Build history of the part. All positions in model axes, mm. A direction names the side the tool comes from. Give positions to 0.01 mm unless a question says otherwise; leave off trailing zeros. Order: outer loops, then holes, each group sorted by start corner. A loop starts at its lowest first (then second) coordinate and runs counter-clockwise, first axis right, second up. Notation, with made-up numbers: (42.25, 58) - (54.25, 58) arc R24 cw to (54.25, 84) - close; hole circle Ø2 at (-1, -33). An arc over 180 degrees is marked (long way). Write each question's results on one line, items separated by ' | '. Start each with the question number.
1) Cut at C-C on x = -892. List the corners of the cut face in (y, z), plus the area to 3 significant figures.
2) Cut at A-A on y = 344.5. List the corners of the cut face in (x, z).
3) Two-plate mould, pull along X, no slides. Class faces 1 (the face through (118.392, 25, -201)), 2 (the face through (650, 50, -277)), 3 (the face through (20, 50, -261)): +X half, -X half, draft (parallel to the pull), parting line (faces both ways), or undercut.
4) Drill centre lines: line 1 along X through (y, z) = (332.5, -290.5); line 2 along Y through (x, z) = (-757.5, -293); line 3 along X through (y, z) = (118.5, -263). Where is each one in solid material? Low to high. Write a range as from..to.
5) Drop flat-ended pins along their axis: pin 1 Ø12 at (x, z) = (9, -253.5) entering from +Y; pin 2 Ø6 at (y, z) = (21.5, -294) entering from +X; pin 3 Ø2 at (y, z) = (275, -258) entering from -X. Give the stop position or say it passes through.
6) Cut at B-B on z = -199.5. List the corners of the cut face in (x, y), plus the area to 3 significant figures.
7) Tool access for faces 4 (the face through (118.392, 272, -276)), 5 (the face through (-131.608, 272, -276)), 6 (the face through (168.392, 272, -276)), 7 (the face through (-81.608, 25, -202)), 8 (the face through (18, 25, -251.508)): list every direction of +Z, -Z, +X, -X, +Y, -Y with a clear straight run to the whole face (end or side of a thin tool).
from build123d import *

# Parameters (mm, degrees)
SKETCH1_W           = 20
SKETCH1_H           = 40
BOSS_EXTRUDE1_DEPTH = 50
SKETCH2_W           = 50
SKETCH2_H           = 50
BOSS_EXTRUDE2_DEPTH = 1000
SKETCH3_W           = 50
SKETCH3_H           = 50
BOSS_EXTRUDE3_DEPTH = 1000
SKETCH4_W           = 50
SKETCH4_H           = 50
BOSS_EXTRUDE4_DEPTH = 450
SKETCH6_W           = 650
SKETCH6_H           = 20
CUT_EXTRUDE2_DEPTH  = 20
SKETCH7_W           = 20
SKETCH7_H           = 450
CUT_EXTRUDE3_DEPTH  = 20


with BuildPart() as part:
    # Sketch1 → Boss-Extrude1 (new body)
    with BuildSketch(Plane(origin=(0, 0, 0), x_dir=(1, 0, 0), z_dir=(0, 1, 0))):
        Polygon((-31.607653806, 251.508316195), (0, 251.508316195), (68.392346194, 251.508316195), (68.392346194, 221.086115448), (68.392346194, 181.086115448), (68.392346194, 151.508316195), (118.392346194, 151.508316195), (118.392346194, 301.508316195), (-81.607653806, 301.508316195), (-81.607653806, 151.508316195), (-31.607653806, 151.508316195), (-31.607653806, 181.086115448), (-31.607653806, 221.086115448), align=None)
        with Locations((-21.607653806, 201.086115448)):
            Rectangle(SKETCH1_W, SKETCH1_H)
        with Locations((58.392346194, 201.086115448)):
            Rectangle(SKETCH1_W, SKETCH1_H)
    extrude(amount=BOSS_EXTRUDE1_DEPTH)

    # Sketch2 → Boss-Extrude2 (add)
    with BuildSketch(Plane(origin=(118.392346194, 0, 0), x_dir=(0, 0, -1), z_dir=(1, 0, 0))):
        with Locations((276.508316195, 25)):
            Rectangle(SKETCH2_W, SKETCH2_H)
    extrude(amount=BOSS_EXTRUDE2_DEPTH)

    # Sketch3 → Boss-Extrude3 (add)
    with BuildSketch(Plane.ZY.offset(81.607653806)):
        with Locations((-276.508316195, 25)):
            Rectangle(SKETCH3_W, SKETCH3_H)
    extrude(amount=BOSS_EXTRUDE3_DEPTH)

    # Sketch4 → Boss-Extrude4 (add)
    with BuildSketch(Plane(origin=(0, 50, 0), x_dir=(1, 0, 0), z_dir=(0, 1, 0))):
        with Locations((-106.607653806, 276.508316195)):
            Rectangle(SKETCH4_W, SKETCH4_H)
        with Locations((143.392346194, 276.508316195)):
            Rectangle(SKETCH4_W, SKETCH4_H)
    extrude(amount=BOSS_EXTRUDE4_DEPTH)

    # Sketch6 → Cut-Extrude2 (cut)
    with BuildSketch(Plane(origin=(0, 0, -301.508316195), x_dir=(-1, 0, 0), z_dir=(0, 0, -1))):
        with Locations((756.607653806, 25)):
            Rectangle(SKETCH6_W, SKETCH6_H)
        with Locations((-793.392346194, 25)):
            Rectangle(SKETCH6_W, SKETCH6_H)
    extrude(amount=-CUT_EXTRUDE2_DEPTH, mode=Mode.SUBTRACT)

    # Sketch7 → Cut-Extrude3 (cut)
    with BuildSketch(Plane(origin=(0, 0, -301.508316195), x_dir=(-1, 0, 0), z_dir=(0, 0, -1))):
        with Locations((-143.392346194, 275)):
            Rectangle(SKETCH7_W, SKETCH7_H)
        with Locations((106.607653806, 275)):
            Rectangle(SKETCH7_W, SKETCH7_H)
    extrude(amount=-CUT_EXTRUDE3_DEPTH, mode=Mode.SUBTRACT)


solid = part.part
Results:
1) outline: (0, -301.51) - (15, -301.51) - (15, -281.51) - (35, -281.51) - (35, -301.51) - (50, -301.51) - (50, -251.51) - (0, -251.51) - close | area: 2,100 mm^2
2) outline: (-131.61, -301.51) - (-116.61, -301.51) - (-116.61, -281.51) - (-96.61, -281.51) - (-96.61, -301.51) - (-81.61, -301.51) - (-81.61, -251.51) - (-131.61, -251.51) - close; (118.39, -301.51) - (133.39, -301.51) - (133.39, -281.51) - (153.39, -281.51) - (153.39, -301.51) - (168.39, -301.51) - (168.39, -251.51) - (118.39, -251.51) - close
3) face 1: +X half | face 2: draft | face 3: undercut
4) line 1: -131.61..-116.61, -96.61..-81.61, 118.39..133.39, 153.39..168.39 | line 2: 0..15, 35..50 | line 3: -131.61..-81.61, 118.39..168.39
5) pin 1: y = 50 | pin 2: x = 468.39 | pin 3: x = -131.61
6) outline: (-81.61, 0) - (-11.61, 0) - (-11.61, 50) - (-81.61, 50) - close; (48.39, 0) - (118.39, 0) - (118.39, 50) - (48.39, 50) - close | area: 7,000 mm^2
7) face 4: +Z, -Z, +Y | face 5: +Z, -Z, -X, +Y | face 6: +Z, -Z, +X, +Y | face 7: +Z, -X, +Y, -Y | face 8: +Y, -Y
